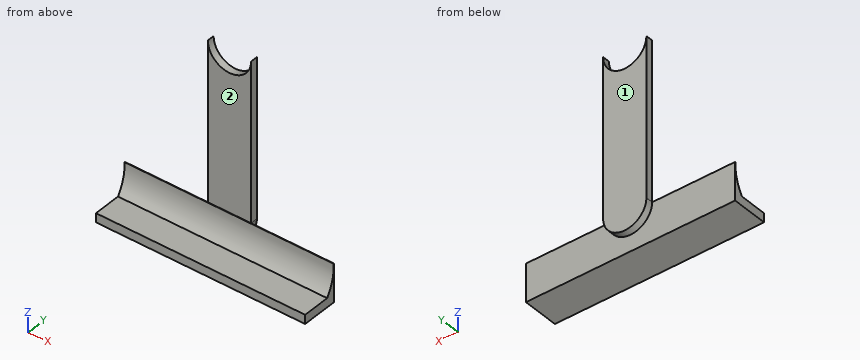
```python
from build123d import *

# Parameters (mm, degrees)
BOX070_W          = 58
BOX070_H          = 10
BOX070_DEPTH      = 2.5
CYLINDER109_R     = 12.5
CYLINDER109_DEPTH = 78
BOX071_W          = 58
BOX071_H          = 10
BOX071_DEPTH      = 10.5
CYLINDER107_W     = 6
CYLINDER107_H     = 2
CYLINDER107_ANGLE = 180
BOX069_W          = 12
BOX069_H          = 2
BOX069_DEPTH      = 44
CYLINDER108_W     = 6
CYLINDER108_H     = 2
CYLINDER108_ANGLE = 180


with BuildPart() as cube059:
    # Box070 → Box070 (new body)
    with BuildSketch(Plane(origin=(68, 24, 21), x_dir=(-1, 0, 0), z_dir=(0, 0, 1))):
        with Locations((29, 5)):
            Rectangle(BOX070_W, BOX070_H)
    extrude(amount=BOX070_DEPTH)


with BuildPart() as cylinder109:
    # Cylinder109 → Cylinder109 (new body)
    with BuildSketch(Plane(origin=(0, 11.4, 30.7), x_dir=(0, 0, -1), z_dir=(1, 0, 0))):
        Circle(CYLINDER109_R)
    extrude(amount=CYLINDER109_DEPTH)


with BuildPart() as fusion042:
    # Box071 → Box071 (new body)
    with BuildSketch(Plane(origin=(68, 24, 21), x_dir=(-1, 0, 0), z_dir=(0, 0, 1))):
        with Locations((29, 5)):
            Rectangle(BOX071_W, BOX071_H)
    extrude(amount=BOX071_DEPTH)

    # Cut056: cut Cylinder109
    add(cylinder109.part, mode=Mode.SUBTRACT)

    # Fusion042: union Cube059
    add(cube059.part)


with BuildPart() as cylinder107:
    # Cylinder107 → Cylinder107 (revolve)
    with BuildSketch(Plane(origin=(39, 26, 75.5), x_dir=(-1, 0, 0), z_dir=(0, 0, 1))):
        with Locations((3, 1)):
            Rectangle(CYLINDER107_W, CYLINDER107_H)
    revolve(axis=Axis((39, 26, 75.5), (0, -1, 0)), revolution_arc=CYLINDER107_ANGLE)


with BuildPart() as cut055:
    # Box069 → Box069 (new body)
    with BuildSketch(Plane(origin=(33, 24, 31.5), x_dir=(1, 0, 0), z_dir=(0, 0, 1))):
        with Locations((6, 1)):
            Rectangle(BOX069_W, BOX069_H)
    extrude(amount=BOX069_DEPTH)

    # Cut055: cut Cylinder107
    add(cylinder107.part, mode=Mode.SUBTRACT)


with BuildPart() as batteryhold001:
    # Cylinder108 → Cylinder108 (revolve)
    with BuildSketch(Plane(origin=(39, 26, 31.5), x_dir=(-1, 0, 0), z_dir=(0, 0, 1))):
        with Locations((3, 1)):
            Rectangle(CYLINDER108_W, CYLINDER108_H)
    revolve(axis=Axis((39, 26, 31.5), (0, -1, 0)), revolution_arc=CYLINDER108_ANGLE)

    # Fusion041: union Cut055
    add(cut055.part)

    # Fusion043: union Fusion042
    add(fusion042.part)


solid = batteryhold001.part
```
The model under review builds one solid part; all positions refer to its coordinate system, in mm. Face numbers are marked on the shaded views. A direction names the side the tool comes from. Round coordinates to 2 decimals unless told otherwise and drop trailing zeros. Order: outer loops, then holes, each group sorted by start corner. A loop starts at its lowest first (then second) coordinate and runs counter-clockwise, first axis right, second up. Notation, with made-up numbers: (42.25, 73) -> (58.25, 73) arc R9 ccw to (58.25, 82) -> close; hole circle Ø7 at (87, 6). An arc over 180 degrees is marked (long way). One line per item, written item: value. Start each with the question number.
Q1. Clearance check with flat-ended pins moving along their axes: pin 1 Ø12 at (x, z) = (56, 58) entering from +Y; pin 2 Ø0.6 at (y, z) = (25, 53) entering from -X; pin 3 Ø12 at (x, z) = (48.5, 39) entering from -Y; pin 4 Ø1 at (y, z) = (25.5, 53) entering from +X. State where each tip first meets the part, or that it passes through.
Q2. Take a section at D-D (x = 42). Write out the cut boundary in (y, z).
Q3. Take a section at A-A (x = 24). Write out the cut boundary in (y, z), and give its area (3 significant figures).
Q4. Take a section at C-C (y = 25.25). Write out the cut boundary in (x, z).
Q5. Take a section at B-B (z = 52.5). Write out the cut boundary in (x, y).
Q6. Machinability: for the marked faces 1 and 2, which of the approach directions +Z, -Z, +X, -X, +Y, -Y give a long, thin tool a straight path to every point of the face, cutting with its end or side? Answer none if there is none.
Q7. Wall thickness on line 1 (Z direction, x = 46, y = 21); line 2 (Y direction, x = 40, z = 46.5); line 3 (X direction, y = 25, z = 39): over which ranges is each line inside the solid? List them lowest first.
Reported:
1. pin 1: passes through
1. pin 2: stops at x = 33
1. pin 3: stops at y = 24
1. pin 4: stops at x = 45
2. outline: (14, 21) -> (24, 21) -> (24, 26.3) -> (26, 26.3) -> (26, 70.3) -> (24, 70.3) -> (24, 31.5) -> (23.87, 31.5) arc R12.5 cw to (21.62, 23.5) -> (14, 23.5) -> close
3. outline: (14, 21) -> (24, 21) -> (24, 31.5) -> (23.87, 31.5) arc R12.5 cw to (21.62, 23.5) -> (14, 23.5) -> close
3. area: 31.1 mm2
4. outline: (33, 31.5) arc R6 ccw to (45, 31.5) -> (45, 75.5) arc R6 cw to (33, 75.5) -> close
5. outline: (33, 24) -> (45, 24) -> (45, 26) -> (33, 26) -> close
6. face 1: +Z, -Z, +X, -X, +Y
6. face 2: +Z, +X, -X, -Y
7. line 1: z = 21 to 23.5
7. line 2: y = 24 to 26
7. line 3: x = 33 to 45
